For this review, take the finished solid that the model builds, in its own axes (mm). Face numbers are marked on the shaded views. A direction names the side the tool comes from. Give positions to 0.01 mm unless a question says otherwise; leave off trailing zeros. Order: outer loops, then holes, each group sorted by start corner. A loop starts at its lowest first (then second) coordinate and runs counter-clockwise, first axis right, second up.
from build123d import *

# Parameters (mm, degrees)
SKETCH2_W           = 45.72
SKETCH2_H           = 55.88
SKETCH2_W_2         = 35.56
SKETCH2_H_2         = 35.56
BOSS_EXTRUDE1_DEPTH = 12.7
SKETCH3_W           = 35.56
SKETCH3_H           = 35.56
BOSS_EXTRUDE2_DEPTH = 4.572
SKETCH4_W           = 35.56
SKETCH4_H           = 35.56
BOSS_EXTRUDE3_DEPTH = 4.572
SKETCH5_W           = 25.4
SKETCH5_H           = 25.4
CUT_EXTRUDE1_DEPTH  = 74.308818023
SKETCH6_R           = 1.7272
CUT_EXTRUDE2_DEPTH  = 74.308818023
SKETCH7_R           = 1.7272
CUT_EXTRUDE3_DEPTH  = 74.308818023
SKETCH8_W           = 1.27
SKETCH8_H           = 55.88
CUT_EXTRUDE4_DEPTH  = 74.308818023


with BuildPart() as part:
    # Sketch2 → Boss-Extrude1 (new body)
    with BuildSketch(Plane.XY):
        with Locations((-22.86, 27.94)):
            Rectangle(SKETCH2_W, SKETCH2_H)
        with Locations((-22.86, 27.94)):
            Rectangle(SKETCH2_W_2, SKETCH2_H_2, mode=Mode.SUBTRACT)
    extrude(amount=BOSS_EXTRUDE1_DEPTH)

    # Sketch3 → Boss-Extrude2 (add)
    with BuildSketch(Plane.XY):
        with Locations((-22.86, 27.94)):
            Rectangle(SKETCH3_W, SKETCH3_H)
    extrude(amount=BOSS_EXTRUDE2_DEPTH)

    # Sketch4 → Boss-Extrude3 (add)
    with BuildSketch(Plane.XY.offset(12.7)):
        with Locations((-22.86, 27.94)):
            Rectangle(SKETCH4_W, SKETCH4_H)
    extrude(amount=-BOSS_EXTRUDE3_DEPTH)

    # Sketch5 → Cut-Extrude1 (cut, through all)
    with BuildSketch(Plane.XY.offset(12.7)):
        with Locations((-22.86, 27.94)):
            Rectangle(SKETCH5_W, SKETCH5_H)
    extrude(amount=-CUT_EXTRUDE1_DEPTH, mode=Mode.SUBTRACT)

    # Sketch6 → Cut-Extrude2 (cut, through all)
    with BuildSketch(Plane.ZY.offset(45.72)):
        with Locations(Location((6.35, 50.8, 0), (0, 0, 270))):
            Circle(SKETCH6_R)
    extrude(amount=-CUT_EXTRUDE2_DEPTH, mode=Mode.SUBTRACT)

    # Sketch7 → Cut-Extrude3 (cut, through all)
    with BuildSketch(Plane.ZY.offset(45.72)):
        with Locations(Location((6.35, 5.08, 0), (0, 0, 270))):
            Circle(SKETCH7_R)
    extrude(amount=-CUT_EXTRUDE3_DEPTH, mode=Mode.SUBTRACT)

    # Sketch8 → Cut-Extrude4 (cut, through all)
    with BuildSketch(Plane.XY.offset(12.7)):
        with Locations((-22.86, 27.94)):
            Rectangle(SKETCH8_W, SKETCH8_H)
    extrude(amount=-CUT_EXTRUDE4_DEPTH, mode=Mode.SUBTRACT)


with BuildPart() as body_2:
    # of the pieces the cut leaves, the one that is kept (cut_extrude4_keep)
    add(part.part.solids().sort_by_distance((-45.72, 55.88, 0))[0])


solid = body_2.part
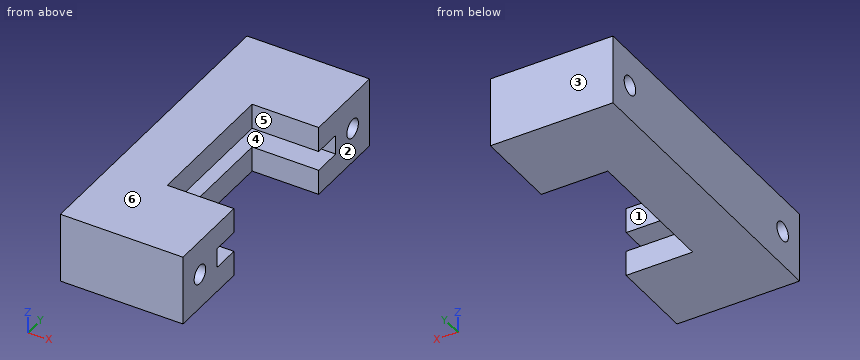
1) Draft analysis for pull direction Y (two halves, no side actions). For the marked faces 1, 2 and 3, state which applies: +Y half, -Y half, draft (parallel to the pull), parting line (faces both ways), or undercut.
Answer sheet:
face 1: undercut
face 2: draft
face 3: +Y half
2) We need section C-C on y = 5.08. Give the boundary of the cut face in (x, z) (3 decimals).
Answer sheet:
outline: (-45.72, 0) - (-23.495, 0) - (-23.495, 4.623) - (-45.72, 4.623) - close; (-45.72, 8.077) - (-23.495, 8.077) - (-23.495, 12.7) - (-45.72, 12.7) - close
3) We need section A-A on x = -25.75. Give the boundary of the cut face in (y, z).
Answer sheet:
outline: (0, 0) - (15.24, 0) - (15.24, 4.57) - (10.16, 4.57) - (10.16, 8.13) - (15.24, 8.13) - (15.24, 12.7) - (0, 12.7) - close; (40.64, 0) - (55.88, 0) - (55.88, 12.7) - (40.64, 12.7) - (40.64, 8.13) - (45.72, 8.13) - (45.72, 4.57) - (40.64, 4.57) - close; hole circle Ø3.45 at (5.08, 6.35); hole circle Ø3.45 at (50.8, 6.35)
4) Tool access review of the marked faces 4, 5 and 6: name each direction out of +Z, -Z, +X, -X, +Y, -Y from which nothing blocks a thin tool from reaching the whole face with its end or side.
Answer sheet:
face 4: +X
face 5: +Z, -Z, +X
face 6: +Z, +X, -X, +Y, -Y
5) To check wall thickness, follow line 1 (Z direction, x = -30.25, y = 5.08); line 2 (Y direction, x = -33.25, z = 5); line 3 (Y direction, x = -35.5, z = 5.5). State the ranges of each line that lie inside material, in increasing order.
Answer sheet:
line 1: z = 0 to 4.62, 8.08 to 12.7
line 2: y = 0 to 4, 6.16 to 10.16, 45.72 to 49.72, 51.88 to 55.88
line 3: y = 0 to 3.58, 6.58 to 10.16, 45.72 to 49.3, 52.3 to 55.88
6) Clearance check with flat-ended pins moving along their axes: pin 1 (5 mm diameter, centred on y = 26.5, z = 2, fed in from +X); pin 2 (10 mm diameter, centred on x = -38, y = 44.5, fed in from -Z); pin 3 (1.8 mm diameter, centred on y = 36, z = 6, fed in from +X). State where each tip first meets the part, or that it passes through.
Answer sheet:
pin 1: stops at x = -35.56
pin 2: stops at z = 0
pin 3: stops at x = -40.64
7) We need section B-B on z = 6.35. Give the boundary of the cut face in (x, y) (3 decimals), then the cut area to 3 significant figures.
Answer sheet:
outline: (-45.72, 0) - (-23.495, 0) - (-23.495, 3.353) - (-45.72, 3.353) - close; (-45.72, 6.807) - (-23.495, 6.807) - (-23.495, 10.16) - (-40.64, 10.16) - (-40.64, 45.72) - (-23.495, 45.72) - (-23.495, 49.073) - (-45.72, 49.073) - close; (-45.72, 52.527) - (-23.495, 52.527) - (-23.495, 55.88) - (-45.72, 55.88) - close
area: 479 mm2
8) We need section D-D on x = -37.75. Give the boundary of the cut face in (y, z).
Answer sheet:
outline: (0, 0) - (55.88, 0) - (55.88, 12.7) - (0, 12.7) - close; hole circle Ø3.45 at (5.08, 6.35); hole (10.16, 4.57) - (45.72, 4.57) - (45.72, 8.13) - (10.16, 8.13) - close; hole circle Ø3.45 at (50.8, 6.35)
